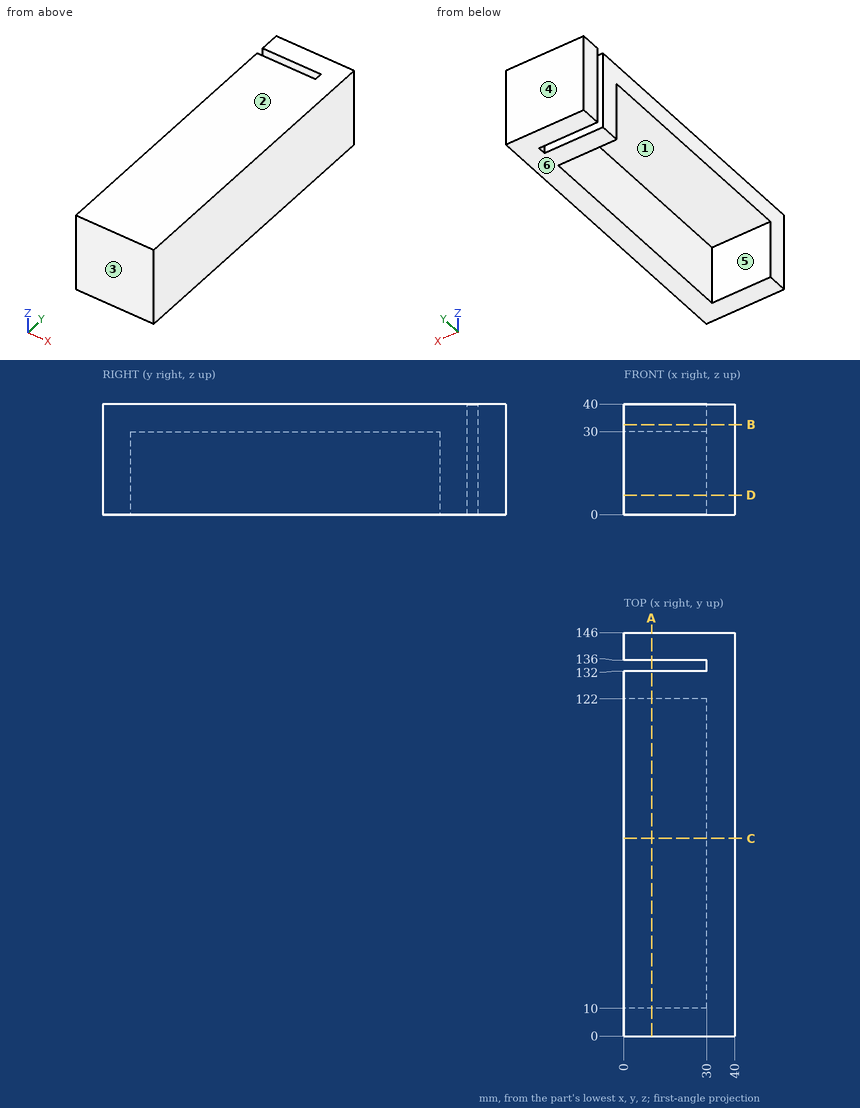
Answer from the drawing. Dimensions are ordinates in mm from the lowest x, y and z of the part. A direction names the side the tool comes from. Coordinates: 2 decimals unless noted, no trailing zeros. Order: outer loops, then holes, each group sorted by start corner. A loop starts at its lowest first (then second) coordinate and runs counter-clockwise, first axis right, second up. Notation, with made-up numbers: M -3.5,41 L 33.5,41 A15 ccw 33.5,60 Z; hole C 26,81.25 d5. An arc over 180 degrees is marked long. Put each result on its own line as item: value. Start each with the question number.
Item 1: For the marked faces 5 and 6, determine the directions among +Z, -Z, +X, -X, +Y, -Y from which every point of the face is accessible in a straight line to the end or side of a thin tool.
Item 2: Section C-C, the plane y = 71.5 is taken. Determine the outline of the cut face in (x, z).
Item 3: Section D-D, the plane z = 7 is taken. Determine the outline of the cut face in (x, y).
Item 4: Consider probe 1 along Y at (x, z) = (27.5, 12); probe 2 along Z at (x, y) = (22.5, 119.5). Determine where each line is inside the solid, lowest interval first. Write a range as [from, to].
Item 5: Section A-A, the plane x = 10 is taken. Determine the outline of the cut face in (y, z), plus the area to 3 significant figures.
Item 6: Given pin 1 Ø2 at (x, y) = (24, 28) entering from -Z; pin 2 Ø1.2 at (y, z) = (134, 19.5) entering from -X, each flat-ended and moving along its own axis, determine where each tip first touches the part or whether it passes through.
Item 7: The mould has two halves that part along Y. Classify the marked faces 1, 2, 3 and 4: +Y half, -Y half, draft (parallel to the pull), parting line (faces both ways), or undercut.
Item 8: Section B-B, the plane z = 32.5 is taken. Determine the outline of the cut face in (x, y).
Computed:
1. face 5: -Z, -X
1. face 6: -Z, +X, -X, +Y, -Y
2. outline: M 0,30 L 30,30 L 30,0 L 40,0 L 40,40 L 0,40 Z
3. outline: M 0,0 L 40,0 L 40,146 L 0,146 L 0,136 L 30,136 L 30,132 L 0,132 L 0,122 L 30,122 L 30,10 L 0,10 Z
4. probe 1: y = [0, 10], [122, 132], [136, 146]
4. probe 2: z = [30, 40]
5. outline: M 0,0 L 10,0 L 10,30 L 122,30 L 122,0 L 132,0 L 132,40 L 0,40 Z; M 136,0 L 146,0 L 146,40 L 136,40 Z
5. area: 2,320 mm2
6. pin 1: stops at z = 30
6. pin 2: stops at x = 30
7. face 1: undercut
7. face 2: draft
7. face 3: -Y half
7. face 4: +Y half
8. outline: M 0,0 L 40,0 L 40,146 L 0,146 L 0,136 L 30,136 L 30,132 L 0,132 Z
